Geometry check sheet. Reference: the model listing, model coordinates, mm. A direction names the side the tool comes from. Give positions to 0.01 mm unless a question says otherwise; leave off trailing zeros. Loops run counter-clockwise (first coordinate to the right, second up) from the corner with the lowest first, then second, coordinate; pieces in that order, holes last.
1. Cross-section at B-B, the plane x = -5. Record the cut outline in (y, z) (3 decimals), plus the area to 3 significant figures.
2. Material ranges on L1, parallel to X at y = 0.25, z = 0.85; L2, parallel to Y at x = -8.25, z = 0.25 (3 decimals); L3, parallel to Y at x = -1.5, z = 1.5 (3 decimals), recorded low to high.
3. Cross-section at A-A, the plane z = 1. Record the cut outline in (x, y) (3 decimals), plus the area to 3 significant figures.
4. Tool access check on faces 1 (the flat face through (-12, 0, 1)), 2 (the flat face through (15, 0, 1)). Record the directions out of +Z, -Z, +X, -X, +Y, -Y that give a thin tool (end or side, any length) a straight path to the whole face; none if there is none.
5. Release check for a two-part mould opening along X. For faces 3 (the flat face through (10, -6, 1.6)), 4 (the cylindrical face through (-14.14, -14.1, 0.79)), 5 (the flat face through (-2.15, -12.5, 0.8)) record: +X half, -X half, draft (parallel to the pull), parting line (faces both ways), or undercut.
6. Cross-section at C-C, the plane y = 8.5. Record the cut outline in (x, z).
from build123d import *

# Parameters (mm, degrees)
F1_DEPTH = 1.6


# Not quite as in the source:
# - a feature names something its author has since deleted; it is built from what else it names


with BuildPart() as f1:
    # F0 (on Top) → F1 (new body)
    with BuildSketch(Plane.XY):
        with BuildLine():
            ThreePointArc((15, 12), (14.1213203436, 14.1213203436), (12, 15))
            Line((12, 15), (-12, 15))
            ThreePointArc((-12, 15), (-14.1213203436, 14.1213203436), (-15, 12))
            Line((-15, 12), (-15, -12))
            ThreePointArc((-15, -12), (-14.1213203436, -14.1213203436), (-12, -15))
            Line((-12, -15), (12, -15))
            ThreePointArc((12, -15), (14.1213203436, -14.1213203436), (15, -12))
            Line((15, -12), (15, 12))
        make_face()
        with BuildLine():
            Line((9.35, -13.025), (-2.15, -13.025))
            Line((-2.15, -13.025), (-2.15, -12.025))
            Line((-2.15, -12.025), (-10, -12.025))
            ThreePointArc((-10, -12.025), (-11.4142135624, -11.4392135624), (-12, -10.025))
            Line((-12, -10.025), (-12, 11))
            ThreePointArc((-12, 11), (-11.7071067812, 11.7071067812), (-11, 12))
            Line((-11, 12), (11, 12))
            ThreePointArc((11, 12), (11.7071067812, 11.7071067812), (12, 11))
            Line((12, 11), (12, -1.525))
            ThreePointArc((12, -1.525), (11.4142135624, -2.9392135624), (10, -3.525))
            Line((10, -3.525), (8.35, -3.525))
            Line((8.35, -3.525), (8.35, -5.525))
            Line((8.35, -5.525), (9.35, -5.525))
            Line((9.35, -5.525), (9.35, -13.025))
        make_face(mode=Mode.SUBTRACT)
    extrude(amount=F1_DEPTH)


solid = f1.part
Result:
1. outline: (-15, 0) - (-12.025, 0) - (-12.025, 1.6) - (-15, 1.6) - close; (12, 0) - (15, 0) - (15, 1.6) - (12, 1.6) - close
1. area: 9.56 mm2
2. L1: x = -15 to -12, 12 to 15
2. L2: y = -15 to -12.025, 12 to 15
2. L3: y = -15 to -13.025, 12 to 15
3. outline: (-15, -12) arc R3 ccw to (-12, -15) - (12, -15) arc R3 ccw to (15, -12) - (15, 12) arc R3 ccw to (12, 15) - (-12, 15) arc R3 ccw to (-15, 12) - close; hole (-12, -10.025) arc R2 ccw to (-10, -12.025) - (-2.15, -12.025) - (-2.15, -13.025) - (9.35, -13.025) - (9.35, -5.525) - (8.35, -5.525) - (8.35, -3.525) - (10, -3.525) arc R2 ccw to (12, -1.525) - (12, 11) arc R1 ccw to (11, 12) - (-11, 12) arc R1 ccw to (-12, 11) - close
3. area: 331 mm2
4. face 1: +Z, -Z
4. face 2: +Z, -Z, +X, +Y, -Y
5. face 3: draft
5. face 4: -X half
5. face 5: undercut
6. outline: (-15, 0) - (-12, 0) - (-12, 1.6) - (-15, 1.6) - close; (12, 0) - (15, 0) - (15, 1.6) - (12, 1.6) - close
